Model file for the job. Use its own axes, mm. Give positions to 0.01 mm unless a question says otherwise; leave off trailing zeros. Loops run counter-clockwise (first coordinate to the right, second up) from the corner with the lowest first, then second, coordinate; pieces in that order, holes last. Notation, with made-up numbers: M -20.75,-24.75 L 18.25,-24.75 A11 ccw 18.25,-12.75 Z; hole C 5.25,-22.5 d10. An arc over 180 degrees is marked long. Use CSV: the item, a comma, the result in double quotes. Start each with the question number.
(1) Slice it at C-C on y = -337. List the corners of the cut face in (x, z).
(2) Wall check: line 1 along Y through (x, z) = (356, 0.75); line 2 along X through (y, z) = (-298, 2.85); line 3 along Y through (x, z) = (449.5, 0.6). Give the ranges that are in metal, low to high. Write a range as from..to.
(3) Slice it at B-B on x = 407. List the corners of the cut face in (y, z), and give its area (3 significant figures).
(4) Slice it at A-A on z = 1.95. State how many separate pieces and enclosed holes the cut face has, and give its area (3 significant figures).
(5) Flat gauge pin, fed straight in: P1, Ø2.5, axis at x = 355.4, y = -280.59, coming from the +Z side. Where does the tip first touch, or does it go through?
```python
from build123d import *

# Parameters (mm, degrees)
SKETCH_1_R      = 1.65
EXTRUDE_1_DEPTH = 4


with BuildPart() as part:
    # 草图1 → 凸台-拉伸1 (new body)
    with BuildSketch(Plane.XY):
        with BuildLine():
            Line((356.978840025, -329.388705272), (424.86396809, -346.465279506))
            ThreePointArc((424.86396809, -346.465279506), (460.82942454, -332.680172491), (460.054173141, -294.171183692))
            Line((460.054173141, -294.171183692), (443.648199748, -271.791638634))
            Line((443.648199748, -271.791638634), (375.763071682, -254.7150644))
            Line((375.763071682, -254.7150644), (350.72066994, -266.668227789))
            ThreePointArc((350.72066994, -266.668227789), (331.816725216, -300.226894433), (356.978840025, -329.388705272))
        make_face()
        with Locations((355.399566463, -280.594209399)):
            Circle(SKETCH_1_R, mode=Mode.SUBTRACT)
        with Locations((381.457813707, -287.149188467)):
            Circle(SKETCH_1_R, mode=Mode.SUBTRACT)
        with Locations((348.844587395, -306.652456643)):
            Circle(SKETCH_1_R, mode=Mode.SUBTRACT)
        with Locations((374.902834639, -313.207435711)):
            Circle(SKETCH_1_R, mode=Mode.SUBTRACT)
        with Locations((423.284694528, -297.670783633)):
            Circle(SKETCH_1_R, mode=Mode.SUBTRACT)
        with Locations((449.342941772, -304.225762701)):
            Circle(SKETCH_1_R, mode=Mode.SUBTRACT)
        with Locations((416.729715461, -323.729030877)):
            Circle(SKETCH_1_R, mode=Mode.SUBTRACT)
        with Locations((442.787962705, -330.284009945)):
            Circle(SKETCH_1_R, mode=Mode.SUBTRACT)
    extrude(amount=EXTRUDE_1_DEPTH)


solid = part.part
```
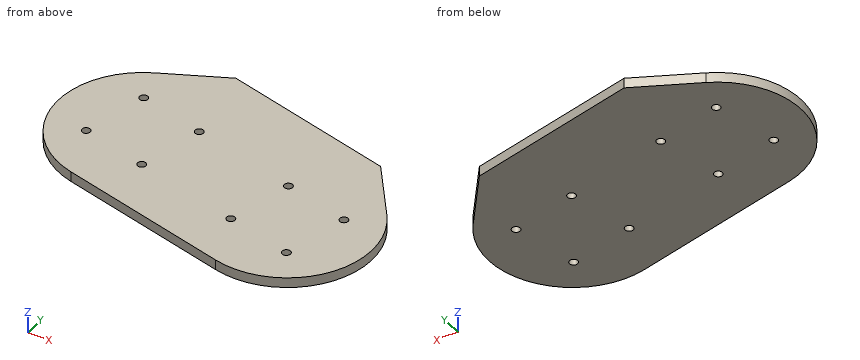
Reply:
1,outline,"M 387.24,0 L 457.37,0 L 457.37,4 L 387.24,4 Z"
2,line 1,"y = -329.13..-282.13, -279.06..-264.15"
2,line 2,"x = 331.67..421.67, 424.9..462.48"
2,line 3,"y = -343.15..-305.87, -302.58..-279.77"
3,outline,"M -341.97,0 L -262.57,0 L -262.57,4 L -341.97,4 Z"
3,area,"318 mm^2"
4,separate pieces,"1"
4,enclosed holes,"8"
4,area,"9,000 mm^2"
5,P1,"passes through"
